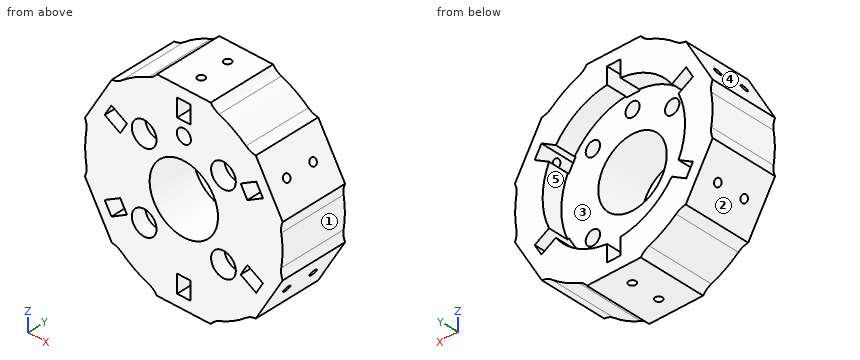
```python
from build123d import *

# Parameters (mm, degrees)
BOSS_EXTRUDE1_DEPTH                          = 30
M3_CLEARANCE_HOLE_PLASTIC_PARTS_ONLY_A_COUNT = 2
M3_CLEARANCE_HOLE_PLASTIC_PARTS_ONLY_A_PITCH = 12.7
WRENCH_START                                 = -5
SKETCH10_W                                   = 5.999999938
SKETCH10_H                                   = 30
WRENCH_CLEARANCE_SLOTS_PLASTIC_PARTS_O_DEPTH = 8
BODY_REVOLVE_PLASTIC_PARTS_ONLY_COUNT        = 6
MOUNTING_SCREWS_D                            = 6.4
MOUNTING_SCREWS_CBORE_D                      = 11
MOUNTING_SCREWS_CBORE_DEPTH                  = 6.5
LOCATING_PIN_D                               = 6.3


with BuildPart() as part:
    # Sketch2 → Boss-Extrude1 (new body)
    with BuildSketch(Plane(origin=(0, 0, 0), x_dir=(1, 0, 0), z_dir=(0, 1, 0))):
        with BuildLine():
            Line((-12, 44), (12, 44))
            ThreePointArc((12, 44), (13.635846147, 42.271481958), (15.707794494, 41.100671432))
            ThreePointArc((15.707794494, 41.100671432), (22, 38.105117767), (27.740328326, 34.153684785))
            ThreePointArc((27.740328326, 34.153684785), (29.790254158, 32.944730144), (32.105117767, 32.392304845))
            Line((32.105117767, 32.392304845), (0, 0))
            Line((0, 0), (-12, 44))
        make_face()
    boss_extrude1 = extrude(amount=-BOSS_EXTRUDE1_DEPTH)

    # Sketch9 → M3 Clearance Hole - Plastic Parts Only (revolve, cut)
    with BuildSketch(Plane(origin=(0, -8.918, -44), x_dir=(0, 1, 0), z_dir=(1, 0, 0))):
        Polygon((0, 0), (0, 10.96138239), (1.6, 10.0000054), (1.6, 0), align=None)
    m3_clearance_hole_plastic_parts_only = revolve(axis=Axis((0, -8.918, -50.35), (0, 0, 1)), mode=Mode.SUBTRACT)

    # M3 Clearance Hole - Plastic Parts Only a: M3 Clearance Hole - Plastic Parts Only ×2
    with Locations(*[(0, -i * M3_CLEARANCE_HOLE_PLASTIC_PARTS_ONLY_A_PITCH, 0) for i in range(1, M3_CLEARANCE_HOLE_PLASTIC_PARTS_ONLY_A_COUNT)]):
        add(m3_clearance_hole_plastic_parts_only, mode=Mode.SUBTRACT)

    # Sketch10 → Wrench Clearance Slots - Plastic Parts Only (cut)
    with BuildSketch(Plane(origin=(0, 0, -44), x_dir=(-1, 0, 0), z_dir=(0, 0, -1)).offset(WRENCH_START)):
        with Locations((0, -15)):
            Rectangle(SKETCH10_W, SKETCH10_H)
    wrench_clearance_slots_plastic_parts_o = extrude(amount=-WRENCH_CLEARANCE_SLOTS_PLASTIC_PARTS_O_DEPTH, mode=Mode.SUBTRACT)

    # Body Revolve - Plastic Parts Only: Boss-Extrude1, M3 Clearance Hole - Plastic Parts Only, Wrench Clearance Slots - Plastic Parts Only ×6 about axis
    body_revolve_plastic_parts_only_axis = Axis((0, 0, 0), (0, 1, 0))
    add([boss_extrude1.rotate(body_revolve_plastic_parts_only_axis, i * 360 / BODY_REVOLVE_PLASTIC_PARTS_ONLY_COUNT) for i in range(1, BODY_REVOLVE_PLASTIC_PARTS_ONLY_COUNT)])
    add([m3_clearance_hole_plastic_parts_only.rotate(body_revolve_plastic_parts_only_axis, i * 360 / BODY_REVOLVE_PLASTIC_PARTS_ONLY_COUNT) for i in range(1, BODY_REVOLVE_PLASTIC_PARTS_ONLY_COUNT)], mode=Mode.SUBTRACT)
    add([wrench_clearance_slots_plastic_parts_o.rotate(body_revolve_plastic_parts_only_axis, i * 360 / BODY_REVOLVE_PLASTIC_PARTS_ONLY_COUNT) for i in range(1, BODY_REVOLVE_PLASTIC_PARTS_ONLY_COUNT)], mode=Mode.SUBTRACT)

    # Body Revolve - Plastic Parts Only copy 1 → Body Revolve - Plastic Parts Only co 2 (revolve, cut)
    with BuildSketch(Plane(origin=(-38.105117767, -21.618, -22), x_dir=(0, 1, 0), z_dir=(0.5000000000000001, 0, -0.8660254037844386))):
        Polygon((0, 0), (0, 10.96138239), (1.6, 10.0000054), (1.6, 0), align=None)
    revolve(axis=Axis((-43.604379081, -21.618, -25.175), (0.8660254037844386, 0, 0.5000000000000001)), mode=Mode.SUBTRACT)

    # Body Revolve - Plastic Parts Only copy 2 → Body Revolve - Plastic Parts Only co 3 (revolve, cut)
    with BuildSketch(Plane(origin=(-38.105117767, -21.618, 22), x_dir=(0, 1, 0), z_dir=(-0.4999999999999998, 0, -0.8660254037844387))):
        Polygon((0, 0), (0, 10.96138239), (1.6, 10.0000054), (1.6, 0), align=None)
    revolve(axis=Axis((-43.604379081, -21.618, 25.175), (0.8660254037844387, 0, -0.4999999999999998)), mode=Mode.SUBTRACT)

    # Body Revolve - Plastic Parts Only copy 3 → Body Revolve - Plastic Parts Only co 4 (revolve, cut)
    with BuildSketch(Plane(origin=(0, -21.618, 44), x_dir=(0, 1, 0), z_dir=(-1, 0, 0))):
        Polygon((0, 0), (0, 10.96138239), (1.6, 10.0000054), (1.6, 0), align=None)
    revolve(axis=Axis((0, -21.618, 50.35), (0, 0, -1)), mode=Mode.SUBTRACT)

    # Body Revolve - Plastic Parts Only copy 4 → Body Revolve - Plastic Parts Only co 5 (revolve, cut)
    with BuildSketch(Plane(origin=(38.105117767, -21.618, 22), x_dir=(0, 1, 0), z_dir=(-0.5000000000000004, 0, 0.8660254037844384))):
        Polygon((0, 0), (0, 10.96138239), (1.6, 10.0000054), (1.6, 0), align=None)
    revolve(axis=Axis((43.604379081, -21.618, 25.175), (-0.8660254037844384, 0, -0.5000000000000004)), mode=Mode.SUBTRACT)

    # Body Revolve - Plastic Parts Only copy 5 → Body Revolve - Plastic Parts Only co 6 (revolve, cut)
    with BuildSketch(Plane(origin=(38.105117767, -21.618, -22), x_dir=(0, 1, 0), z_dir=(0.5000000000000001, 0, 0.8660254037844386))):
        Polygon((0, 0), (0, 10.96138239), (1.6, 10.0000054), (1.6, 0), align=None)
    revolve(axis=Axis((43.604379081, -21.618, -25.175), (-0.8660254037844386, 0, 0.5000000000000001)), mode=Mode.SUBTRACT)

    # Sketch3 → End of Arm Flange Clearance (revolve, cut)
    with BuildSketch(Plane.XY, mode=Mode.PRIVATE) as end_of_arm_flange_clearance_sk:
        Polygon((0, 0), (0, -30), (15.25, -30), (15.25, -9), (31.75, -9), (31.75, 0), align=None)
    revolve(end_of_arm_flange_clearance_sk.sketch.rotate(Axis((0, -948.680059029, 0), (0, 1, 0)), 90), axis=Axis((0, -948.680059029, 0), (0, 1, 0)), mode=Mode.SUBTRACT)

    # Mounting Screws (through all)
    with Locations(Plane(origin=(0, -30, 0), x_dir=(-1, 0, 0), z_dir=(0, -1, 0))):
        with Locations((-17.67766953, -17.67766953), (-17.67766953, 17.67766953), (17.67766953, 17.67766953), (17.67766953, -17.67766953)):
            CounterBoreHole(MOUNTING_SCREWS_D / 2, MOUNTING_SCREWS_CBORE_D / 2, MOUNTING_SCREWS_CBORE_DEPTH)

    # Locating Pin (through all)
    with Locations(Plane(origin=(0, -30, 0), x_dir=(-1, 0, 0), z_dir=(0, -1, 0))):
        with Locations((0, -25)):
            Hole(LOCATING_PIN_D / 2)


solid = part.part
```
The model under review builds one solid part; all positions refer to its coordinate system, in mm. Face numbers are marked on the shaded views. A direction names the side the tool comes from. Give positions to 0.01 mm unless a question says otherwise; leave off trailing zeros. Write each loop counter-clockwise with the first axis right and the second up, starting at its lowest first coordinate (ties: lowest second). Pieces come first, ordered by that corner, then holes. Notation, with made-up numbers: M 14,41 L 56,41 A21 cw 56,60 Z; hole C 21.25,63.5 d10. An arc over 180 degrees is marked long. Answer in a Markdown table with one row per item.
Item 1: Tool access review of the marked faces 4 and 5: name each direction out of +Z, -Z, +X, -X, +Y, -Y from which nothing blocks a thin tool from reaching the whole face with its end or side.
Check sheet entries:
| item | result |
|---|---|
| face 4 | +Z, -X, +Y, -Y |
| face 5 | +Y |
Item 2: For P1, Ø8, axis at x = -16, z = -21.5, coming from the +Y side; P2, Ø6.5, axis at y = -17.5, z = -33.5, coming from the +X side; P3, Ø2, axis at x = 0.5, z = 26, coming from the +Y side; P4, Ø3, axis at x = 0, y = -8.918, coming from the +Z side, all flat-tipped, find the tip position at first contact; note any pin that passes through.
Check sheet entries:
| item | result |
|---|---|
| P1 | y = -9 |
| P2 | x = 33.34 |
| P3 | through |
| P4 | z = 31 |
Item 3: Add section D-D on z = 25. Give the boundary of the cut face in (x, y).
Check sheet entries:
| item | result |
|---|---|
| outline | M -36.37,-30 L -3.15,-30 L -3.15,-9 L -19.57,-9 L -19.57,0 L -36.37,0 Z; M 3.15,-30 L 36.37,-30 L 36.37,0 L 19.57,0 L 19.57,-9 L 3.15,-9 Z |
Item 4: For line 1 along Y through (x, z) = (0, 40); line 2 along Z through (x, y) = (37, -20.5); line 3 along X through (y, z) = (-14, 21.5), list the stretches that pass through material, from the lowest coordinate up.
Check sheet entries:
| item | result |
|---|---|
| line 1 | -30 to -23.22, -20.02 to -10.52, -7.32 to 0 |
| line 2 | -23.91 to -22.68, -20.04 to 20.04, 22.68 to 23.91 |
| line 3 | -38.39 to -32.62, -31.24 to 31.24, 32.62 to 38.39 |
Item 5: Draft analysis for pull direction X (two halves, no side actions). For the marked faces 1, 2 and 3, state which applies: +X half, -X half, draft (parallel to the pull), parting line (faces both ways), or undercut.
Check sheet entries:
| item | result |
|---|---|
| face 1 | +X half |
| face 2 | -X half |
| face 3 | undercut |
Item 6: Add section C-C on x = 0. State how many separate pieces and enclosed holes the cut face has, plus the area to 3 significant figures.
Check sheet entries:
| item | result |
|---|---|
| separate pieces | 9 |
| enclosed holes | 0 |
| area | 765 mm2 |
Item 7: Add section A-A on z = 0. Give the boundary of the cut face in (x, y), plus the area to 3 significant figures.
Check sheet entries:
| item | result |
|---|---|
| outline | M -44,-30 L -15.25,-30 L -15.25,-9 L -31.75,-9 L -31.75,0 L -44,0 Z; M 15.25,-30 L 44,-30 L 44,0 L 31.75,0 L 31.75,-9 L 15.25,-9 Z |
| area | 1,430 mm2 |
Item 8: Add section B-B on x = -17.5. Give the boundary of the cut face in (y, z).
Check sheet entries:
| item | result |
|---|---|
| outline | M -30,-40.37 L 0,-40.37 L 0,-26.49 L -9,-26.49 L -9,-20.87 L -23.5,-20.87 L -23.5,-23.17 L -30,-23.17 Z; M -30,-12.18 L -23.5,-12.18 L -23.5,-14.48 L -9,-14.48 L -9,14.48 L -23.5,14.48 L -23.5,12.18 L -30,12.18 Z; M -30,23.17 L -23.5,23.17 L -23.5,20.87 L -9,20.87 L -9,26.49 L 0,26.49 L 0,40.37 L -30,40.37 Z |
